For this review, take the finished solid that the model builds, in its own axes (mm). A direction names the side the tool comes from. Coordinates: 2 decimals unless noted, no trailing zeros. Order: outer loops, then holes, each group sorted by start corner. A loop starts at its lowest first (then second) coordinate and runs counter-clockwise, first axis right, second up. Notation, with made-up numbers: (-19.5, -17.5) -> (9.5, -17.5) arc R10 ccw to (9.5, -10.5) -> close; hole circle Ø1 at (16.5, 6.5). An arc over 180 degrees is marked (long way). Answer as a JSON object with one key per item and string values. Group by question number.
1) Machinability: for faces 1 (the flat face through (-3, -51.75, 173)), 2 (the flat face through (7, -46.75, 248)), which of the approach directions +Z, -Z, +X, -X, +Y, -Y give a long, thin tool a straight path to every point of the face, cutting with its end or side? Answer none if there is none.
2) Add section A-A, the plane z = 300. Write out the cut boundary in (x, y), then the cut area to 3 significant figures.
3) Wall thickness on L1, parallel to X at y = -48.85, z = 300; L2, parallel to X at y = -50.45, z = 310.5; L3, parallel to X at y = -50.45, z = 170 (3 decimals): over which ranges is each line inside the solid? List them lowest first.
4) For pin 1 (1 mm diameter, centred on y = -48, z = 331, fed in from +X), flat-tipped, find the tip position at first contact; note if it passes through.
5) Add section D-D, the plane x = 12.5. Write out the cut boundary in (y, z).
6) Draft analysis for pull direction X (two halves, no side actions). For faces 3 (the flat face through (35, -50, 251)), 4 (the cylindrical face through (-0.77, -49.79, 364.99)), 5 (the cylindrical face through (0.099, -49.792, 308.252)), state which applies: +X half, -X half, draft (parallel to the pull), parting line (faces both ways), or undercut.
7) Add section B-B, the plane y = -47.8. Write out the cut boundary in (x, z) (3 decimals), then the cut area to 3 significant figures.
8) Add section C-C, the plane z = 349.5. Write out the cut boundary in (x, y), then the cut area to 3 significant figures.
from build123d import *

# Parameters (mm, degrees)
PLACA_START                   = -52.75
SK_PLACA_W                    = 70
SK_PLACA_H                    = 160
PLACA_DEPTH                   = 6
EXTREMOS_START                = -52.75
SK_EXTREMOS_R                 = 35
EXTREMOS_DEPTH                = 6
PASANTES_M4_SEPARADORES_START = -52.75
SK_PASANTES_M4_SEPARADORES_R  = 2.25
PASANTES_M4_SEPARADORES_DEPTH = 6
ALOJAMIENTO_696ZZ_START       = -51.75
SK_ALOJAMIENTO_696ZZ_R        = 7.475
ALOJAMIENTO_696ZZ_DEPTH       = 5
PASO_EXTRACTOR_START          = -52.75
SK_PASO_EXTRACTOR_R           = 4
PASO_EXTRACTOR_DEPTH          = 1
PASANTES_M4_EJEFALSO_J3_START = -52.75
SK_PASANTES_M4_EJEFALSO_J3_R  = 2.25
PASANTES_M4_EJEFALSO_J3_DEPTH = 6


with BuildPart() as part:
    # Sk_Placa → Placa (new body)
    with BuildSketch(Plane(origin=(0, 0, 0), x_dir=(1, 0, 0), z_dir=(0, 1, 0)).offset(PLACA_START)):
        with Locations((0, -250)):
            Rectangle(SK_PLACA_W, SK_PLACA_H)
    extrude(amount=PLACA_DEPTH)

    # Sk_Extremos → Extremos (add)
    with BuildSketch(Plane(origin=(0, 0, 0), x_dir=(1, 0, 0), z_dir=(0, 1, 0)).offset(EXTREMOS_START)):
        with Locations((0, -170)):
            Circle(SK_EXTREMOS_R)
        with Locations((0, -330)):
            Circle(SK_EXTREMOS_R)
    extrude(amount=EXTREMOS_DEPTH)

    # Sk_Pasantes_M4_separadores → Pasantes_M4_separadores (cut)
    with BuildSketch(Plane(origin=(0, 0, 0), x_dir=(1, 0, 0), z_dir=(0, 1, 0)).offset(PASANTES_M4_SEPARADORES_START)):
        with Locations(Location((0, -250, 0), (0, 0, 270))):
            Circle(SK_PASANTES_M4_SEPARADORES_R)
        with Locations(Location((-22, -300, 0), (0, 0, 270))):
            Circle(SK_PASANTES_M4_SEPARADORES_R)
        with Locations(Location((22, -300, 0), (0, 0, 270))):
            Circle(SK_PASANTES_M4_SEPARADORES_R)
    extrude(amount=PASANTES_M4_SEPARADORES_DEPTH, mode=Mode.SUBTRACT)

    # Sk_Alojamiento_696ZZ → Alojamiento_696ZZ (cut)
    with BuildSketch(Plane(origin=(0, 0, 0), x_dir=(1, 0, 0), z_dir=(0, 1, 0)).offset(ALOJAMIENTO_696ZZ_START)):
        with Locations(Location((0, -170, 0), (0, 0, 270))):
            Circle(SK_ALOJAMIENTO_696ZZ_R)
    extrude(amount=ALOJAMIENTO_696ZZ_DEPTH, mode=Mode.SUBTRACT)

    # Sk_Paso_extractor → Paso_extractor (cut)
    with BuildSketch(Plane(origin=(0, 0, 0), x_dir=(1, 0, 0), z_dir=(0, 1, 0)).offset(PASO_EXTRACTOR_START)):
        with Locations(Location((0, -170, 0), (0, 0, 270))):
            Circle(SK_PASO_EXTRACTOR_R)
    extrude(amount=PASO_EXTRACTOR_DEPTH, mode=Mode.SUBTRACT)

    # Sk_Pasantes_M4_ejefalso_J3 → Pasantes_M4_ejefalso_J3 (cut)
    with BuildSketch(Plane(origin=(0, 0, 0), x_dir=(1, 0, 0), z_dir=(0, 1, 0)).offset(PASANTES_M4_EJEFALSO_J3_START)):
        with Locations(Location((0, -310.5, 0), (0, 0, 270))):
            Circle(SK_PASANTES_M4_EJEFALSO_J3_R)
        with Locations(Location((0, -349.5, 0), (0, 0, 270))):
            Circle(SK_PASANTES_M4_EJEFALSO_J3_R)
    extrude(amount=PASANTES_M4_EJEFALSO_J3_DEPTH, mode=Mode.SUBTRACT)


solid = part.part
Output values:
{
 "1": {"face 1": "+Y", "face 2": "+Z, -Z, +X, -X, +Y"},
 "2": {"outline": "(-35, -52.75) -> (-24.25, -52.75) -> (-24.25, -46.75) -> (-35, -46.75) -> close; (-19.75, -52.75) -> (19.75, -52.75) -> (19.75, -46.75) -> (-19.75, -46.75) -> close; (24.25, -52.75) -> (35, -52.75) -> (35, -46.75) -> (24.25, -46.75) -> close", "area": "366 mm²"},
 "3": {"L1": "x = -35 to -24.25, -19.75 to 19.75, 24.25 to 35", "L2": "x = -35 to -2.25, 2.25 to 35", "L3": "x = -35 to -7.475, 7.475 to 35"},
 "4": {"pin 1": "stops at x = 35"},
 "5": {"outline": "(-52.75, 137.31) -> (-46.75, 137.31) -> (-46.75, 362.69) -> (-52.75, 362.69) -> close"},
 "6": {"face 3": "+X half", "face 4": "parting line", "face 5": "undercut"},
 "7": {"outline": "(-35, 170) arc R35 ccw to (35, 170) -> (35, 330) arc R35 ccw to (-35, 330) -> close; hole circle Ø4.5 at (-22, 300); hole circle Ø14.95 at (0, 170); hole circle Ø4.5 at (0, 250); hole circle Ø4.5 at (0, 310.5); hole circle Ø4.5 at (0, 349.5); hole circle Ø4.5 at (22, 300)", "area": "14,800 mm²"},
 "8": {"outline": "(-29.06, -52.75) -> (-2.25, -52.75) -> (-2.25, -46.75) -> (-29.06, -46.75) -> close; (2.25, -52.75) -> (29.06, -52.75) -> (29.06, -46.75) -> (2.25, -46.75) -> close", "area": "322 mm²"}
}
